from build123d import *

# Parameters (mm, degrees)
SKETCH1_W          = 25.4
SKETCH1_H          = 152.4
EXTRUDE1_DEPTH     = 3.175
SKETCH3_W          = 3.175
SKETCH3_H          = 6.35
CUT_EXTRUDE1_DEPTH = 3.175
LPATTERN1_COUNT    = 2
LPATTERN1_PITCH    = 146.05
SKETCH4_W          = 3.175
SKETCH4_H          = 12.7
CUT_EXTRUDE2_DEPTH = 3.175
LPATTERN2_COUNT    = 5
LPATTERN2_PITCH    = 25.4
SKETCH5_W          = 12.7
SKETCH5_H          = 3.175
CUT_EXTRUDE3_DEPTH = 3.175
SKETCH6_W          = 6.35
SKETCH6_H          = 3.175
CUT_EXTRUDE4_DEPTH = 3.175
LPATTERN3_COUNT    = 2
LPATTERN3_PITCH    = 19.05


with BuildPart() as part:
    # Sketch1 → Extrude1 (new body)
    with BuildSketch(Plane.XY):
        with Locations((12.7, 76.2)):
            Rectangle(SKETCH1_W, SKETCH1_H)
    extrude(amount=EXTRUDE1_DEPTH)

    # Sketch3 → Cut-Extrude1 (cut)
    with BuildSketch(Plane.XY.offset(3.175)):
        with Locations((23.8125, 149.225)):
            Rectangle(SKETCH3_W, SKETCH3_H)
    cut_extrude1 = extrude(amount=-CUT_EXTRUDE1_DEPTH, mode=Mode.SUBTRACT)

    # LPattern1: Cut-Extrude1 ×2
    with Locations(*[(0, -i * LPATTERN1_PITCH, 0) for i in range(1, LPATTERN1_COUNT)]):
        add(cut_extrude1, mode=Mode.SUBTRACT)

    # Sketch4 → Cut-Extrude2 (cut)
    with BuildSketch(Plane.XY.offset(3.175)):
        with Locations((23.8125, 127)):
            Rectangle(SKETCH4_W, SKETCH4_H)
    cut_extrude2 = extrude(amount=-CUT_EXTRUDE2_DEPTH, mode=Mode.SUBTRACT)

    # LPattern2: Cut-Extrude2 ×5
    with Locations(*[(0, -i * LPATTERN2_PITCH, 0) for i in range(1, LPATTERN2_COUNT)]):
        add(cut_extrude2, mode=Mode.SUBTRACT)

    # Sketch5 → Cut-Extrude3 (cut)
    with BuildSketch(Plane.XY.offset(3.175)):
        with Locations((12.7, 1.5875)):
            Rectangle(SKETCH5_W, SKETCH5_H)
    extrude(amount=-CUT_EXTRUDE3_DEPTH, mode=Mode.SUBTRACT)

    # Sketch6 → Cut-Extrude4 (cut)
    with BuildSketch(Plane.XY.offset(3.175)):
        with Locations((3.175, 150.8125)):
            Rectangle(SKETCH6_W, SKETCH6_H)
    cut_extrude4 = extrude(amount=-CUT_EXTRUDE4_DEPTH, mode=Mode.SUBTRACT)

    # LPattern3: Cut-Extrude4 ×2
    with Locations(*[(i * LPATTERN3_PITCH, 0, 0) for i in range(1, LPATTERN3_COUNT)]):
        add(cut_extrude4, mode=Mode.SUBTRACT)


solid = part.part
Can you work these out from the model? Positions are in its coordinate system, mm. A direction names the side the tool comes from. Round coordinates to 2 decimals unless told otherwise and drop trailing zeros. Loops run counter-clockwise (first coordinate to the right, second up) from the corner with the lowest first, then second, coordinate; pieces in that order, holes last. Notation, with made-up numbers: (58, 61.5) - (76, 61.5) arc R16 cw to (76, 76.5) - close; hole circle Ø5 at (41, 62). An arc over 180 degrees is marked (long way). Use CSV: the item, a comma, the result in double quotes. Start each with the question number.
1) If we section it at A-A on x = 24: Write out the boundary of the cut face in (y, z) (3 decimals), plus the area to 3 significant figures.
2) If we section it at C-C on x = 11: Write out the boundary of the cut face in (y, z) (3 decimals), plus the area to 3 significant figures.
3) For pin 1 Ø1 at (y, z) = (2, 1) entering from +X (3 decimals); pin 2 Ø1 at (y, z) = (151.5, 1) entering from +X; pin 3 Ø3 at (x, y) = (7.5, 79.5) entering from -Z; pin 4 Ø1.6 at (x, z) = (24.5, 1.5) entering from -Y, each with a flat end and sliding along its axis, tell me the tip position at first contact or that it passes through.
4) For faces 1 (the flat face through (13, 3.175, 2)), 2 (the flat face through (24, 146.05, 2)), 3 (the flat face through (22.225, 76, 2)), 4 (the flat face through (25.4, 140, 2)), 5 (the flat face through (6.35, 151, 2)), which set-ups out of +Z, -Z, +X, -X, +Y, -Y let a thin tool reach every point of the face, with its end or its side?
5) If we section it at B-B on y = 27.5: Write out the boundary of the cut face in (x, z) (3 decimals), plus the area to 3 significant figures.
6) Please list where these lines run through material, in increasing order: probe 1 along Y at (x, z) = (24.25, 0.8); probe 2 along X at (y, z) = (50, 2.5) (3 decimals); probe 3 along Y at (x, z) = (14, 2) (3 decimals). Write a range as [from, to].
7) We'd pull the mould along Y, two halves only. Please class faces 6 (the flat face through (24, 107.95, 2)), 7 (the flat face through (24, 19.05, 2)), 8 (the flat face through (13, 152.4, 2)), 9 (the flat face through (22.225, 3, 2)): released by +Y, released by -Y, zero draft, split by the parting line, or undercut.
Geometry results:
1,outline,"(6.35, 0) - (19.05, 0) - (19.05, 3.175) - (6.35, 3.175) - close; (31.75, 0) - (44.45, 0) - (44.45, 3.175) - (31.75, 3.175) - close; (57.15, 0) - (69.85, 0) - (69.85, 3.175) - (57.15, 3.175) - close; (82.55, 0) - (95.25, 0) - (95.25, 3.175) - (82.55, 3.175) - close; (107.95, 0) - (120.65, 0) - (120.65, 3.175) - (107.95, 3.175) - close; (133.35, 0) - (146.05, 0) - (146.05, 3.175) - (133.35, 3.175) - close"
1,area,"242 mm2"
2,outline,"(3.175, 0) - (152.4, 0) - (152.4, 3.175) - (3.175, 3.175) - close"
2,area,"474 mm2"
3,pin 1,"stops at x = 22.225"
3,pin 2,"stops at x = 19.05"
3,pin 3,"stops at z = 0"
3,pin 4,"stops at y = 6.35"
4,face 1,"+Z, -Z, -Y"
4,face 2,"+Z, -Z, +X, +Y"
4,face 3,"+Z, -Z, +X"
4,face 4,"+Z, -Z, +X, +Y, -Y"
4,face 5,"+Z, -Z, -X, +Y"
5,outline,"(0, 0) - (22.225, 0) - (22.225, 3.175) - (0, 3.175) - close"
5,area,"70.6 mm2"
6,probe 1,"y = [6.35, 19.05], [31.75, 44.45], [57.15, 69.85], [82.55, 95.25], [107.95, 120.65], [133.35, 146.05]"
6,probe 2,"x = [0, 22.225]"
6,probe 3,"y = [3.175, 152.4]"
7,face 6,"undercut"
7,face 7,"undercut"
7,face 8,"released by +Y"
7,face 9,"zero draft"
